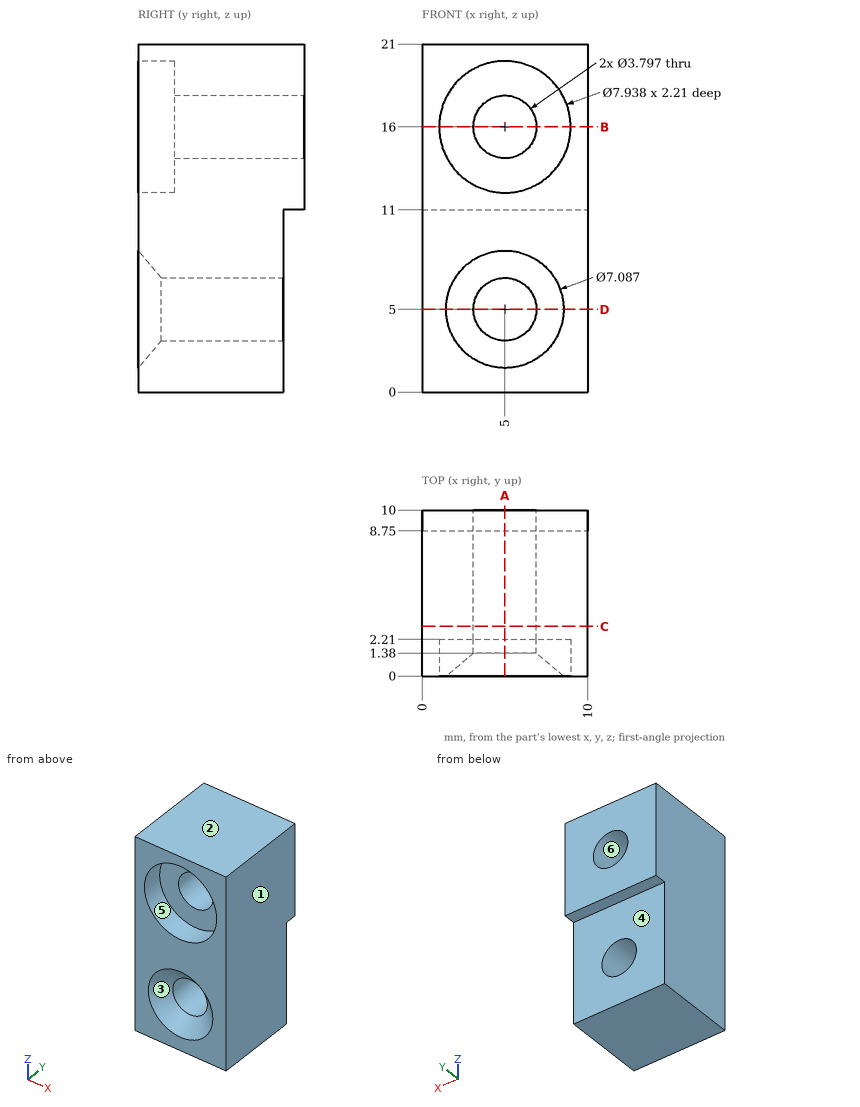
Study the drawing (mm; zero at the part's minimum x, y, z) and answer. A direction names the side the tool comes from. Give positions to 0.01 mm unless a question says otherwise; leave off trailing zeros. Write each loop counter-clockwise with the first axis right and the second up, starting at its lowest first coordinate (ties: lowest second). Pieces come first, ordered by that corner, then holes. Notation, with made-up numbers: (21.25, 55) - (69.25, 55) arc R8 cw to (69.25, 68) - close; hole circle Ø10 at (-34.75, 55). An arc over 180 degrees is marked (long way). Use a Markdown table: item, result.
1. For a pull along Z with two mould halves and no side action, classify the marked faces 1, 2 and 3 as released by +Z, released by -Z, zero draft, split by the parting line, or undercut.
Values follow:
| item | result |
|---|---|
| face 1 | zero draft |
| face 2 | released by +Z |
| face 3 | undercut |
2. Section A-A on x = 5 is taken. Write down the section's boundary in (y, z), plus the area to 3 significant figures.
Values follow:
| item | result |
|---|---|
| outline | (0, 0) - (8.75, 0) - (8.75, 3.1) - (1.38, 3.1) - (0, 1.46) - close; (0, 8.54) - (1.38, 6.9) - (8.75, 6.9) - (8.75, 11) - (10, 11) - (10, 14.1) - (2.21, 14.1) - (2.21, 12.03) - (0, 12.03) - close; (0, 19.97) - (2.21, 19.97) - (2.21, 17.9) - (10, 17.9) - (10, 21) - (0, 21) - close |
| area | 114 mm² |
3. Section D-D on z = 5 is taken. Write down the section's boundary in (x, y).
Values follow:
| item | result |
|---|---|
| outline | (0, 0) - (1.46, 0) - (3.1, 1.38) - (3.1, 8.75) - (0, 8.75) - close; (6.9, 1.38) - (8.54, 0) - (10, 0) - (10, 8.75) - (6.9, 8.75) - close |
4. Section C-C on y = 3 is taken. Write down the section's boundary in (x, z).
Values follow:
| item | result |
|---|---|
| outline | (0, 0) - (10, 0) - (10, 21) - (0, 21) - close; hole circle Ø3.8 at (5, 5); hole circle Ø3.8 at (5, 16) |
5. Section B-B on z = 16 is taken. Write down the section's boundary in (x, y).
Values follow:
| item | result |
|---|---|
| outline | (0, 0) - (1.03, 0) - (1.03, 2.21) - (3.1, 2.21) - (3.1, 10) - (0, 10) - close; (6.9, 2.21) - (8.97, 2.21) - (8.97, 0) - (10, 0) - (10, 10) - (6.9, 10) - close |
6. Find the intervals of material crossed by probe 1 along Z at (x, y) = (5, 5.75); probe 2 along Z at (x, y) = (6.5, 8.5) (1 decimal); probe 3 along X at (y, z) = (7.5, 16), in increasing order. Write a range as from..to.
Values follow:
| item | result |
|---|---|
| probe 1 | z = 0..3.1, 6.9..14.1, 17.9..21 |
| probe 2 | z = 0..3.8, 6.2..14.8, 17.2..21 |
| probe 3 | x = 0..3.1, 6.9..10 |
7. A tool of negligible diameter and unlimited length cuts with its end or side. For the marked faces 4, 5 and 6, from which of +Z, -Z, +X, -X, +Y, -Y can it reach the whole face along a straight path? Write none if from no direction.
Values follow:
| item | result |
|---|---|
| face 4 | -Z, +X, -X, +Y |
| face 5 | -Y |
| face 6 | +Y, -Y |
8. Each of these flat-tipped pins is pushed along its axis until it touches: P1, Ø6, axis at x = 5, z = 16, coming from the -Y side; P2, Ø4.5, axis at x = 5, z = 5, coming from the -Y side (1 decimal); P3, Ø0.6, axis at x = 3.5, y = 9.5, coming from the -Z side. Where does it stop, or does it pass through?
Values follow:
| item | result |
|---|---|
| P1 | stops at y = 2.21 |
| P2 | stops at y = 1.1 |
| P3 | stops at z = 11 |
